Could you check a few things on this model? Use its own coordinates, in mm. A direction names the side the tool comes from. Coordinates: 2 decimals unless noted, no trailing zeros. Write each loop counter-clockwise with the first axis right and the second up, starting at its lowest first coordinate (ties: lowest second). Pieces come first, ordered by that corner, then holes. Notation, with made-up numbers: M 31,21.25 L 60,21.25 A27 ccw 60,53.25 Z; hole C 21.5,13.5 d4. An arc over 180 degrees is marked long. Answer as CSV lines item,"result". Start each with the question number.
Item 1: On a 3-axis mill with a long thin cutter (end or side, diameter ignored), from which of +Z, -Z, +X, -X, +Y, -Y can I reach the whole of each face in a straight line? I mean faces 1 (the cylindrical face through (-8.107, -8.156, 0.37)), 2 (the flat face through (8.475, 11, -4)), 3 (the cylindrical face through (6.31, 10.79, -2.46)). Say none if no direction works.
Item 2: We'd pull the mould along X, two halves only. Please class faces 4 (the flat face through (-8.475, 11, -4)), 5 (the flat face through (0, 9.45, -4)), 6 (the cylindrical face through (-8.156, 8.107, 0.37)), 7 (the cylindrical face through (-0.1, 10, 0.4)): +X half, -X half, draft (parallel to the pull), parting line (faces both ways), or undercut.
Item 3: Suppose I cut it at B-B, the plane z = -3.5. Write out the boundary of the cut face in (x, y) (3 decimals), and give its area (3 significant figures).
Item 4: I'm going to push flat-ended pins straight in: P1, Ø2, axis at x = 6.5, y = 7.5, coming from the -Z side; P2, Ø1, axis at x = 2, z = -3.5, coming from the -Y side; P3, Ø1.3, axis at y = 11, z = -3, coming from the +X side (3 decimals); P4, Ø6, axis at x = -3.5, y = -3.5, coming from the +Z side. Where does each tip first touch, or does it pass through?
Item 5: Suppose I cut it at A-A, the plane x = 0. Write out the boundary of the cut face in (y, z).
Item 6: Suppose I cut it at C-C, the plane y = 2.75. Write out the boundary of the cut face in (x, z) (3 decimals).
Item 7: If I drill on line 1 along Y through (x, z) = (0, -1); line 2 along X through (y, z) = (0, -1.2) (3 decimals); line 3 along Z through (x, y) = (6.5, 7), over which ranges is the centre line in solid material (lowest first)? Write a range as [from, to].
Item 8: Suppose I cut it at D-D, the plane z = 0.5. Write out the boundary of the cut face in (x, y) (3 decimals).
```python
from build123d import *

# Parameters (mm, degrees)
F0_W     = 20.15
F0_H     = 22.85
F1_DEPTH = 0.75
F2_W     = 20.15
F2_H     = 22.85
F2_R     = 8.5
F3_DEPTH = 2.15
F4_W     = 16.95
F4_H     = 2.65
F5_DEPTH = 3.45
F6_R     = 1.05
F7_DEPTH = 22.851


with BuildPart() as f1:
    # F0 (on Top) → F1 (new body)
    with BuildSketch(Plane.XY):
        with Locations((0, 0.675)):
            Rectangle(F0_W, F0_H)
        with BuildLine():
            ThreePointArc((8.049191, 5.933845), (9.499787, 3.123147), (10, 0))
            ThreePointArc((10, 0), (9.499787, -3.123147), (8.049191, -5.933845))
            ThreePointArc((8.049191, -5.933845), (8.43437, -6.445442), (8.571068, -7.071068))
            ThreePointArc((8.571068, -7.071068), (7.592684, -8.477452), (5.933845, -8.049191))
            ThreePointArc((5.933845, -8.049191), (0, -10), (-5.933845, -8.049191))
            ThreePointArc((-5.933845, -8.049191), (-8.131728, -8.131728), (-8.049191, -5.933845))
            ThreePointArc((-8.049191, -5.933845), (-10, 0), (-8.049191, 5.933845))
            ThreePointArc((-8.049191, 5.933845), (-8.131728, 8.131728), (-5.933845, 8.049191))
            ThreePointArc((-5.933845, 8.049191), (0, 10), (5.933845, 8.049191))
            ThreePointArc((5.933845, 8.049191), (7.592684, 8.477452), (8.571068, 7.071068))
            ThreePointArc((8.571068, 7.071068), (8.43437, 6.445442), (8.049191, 5.933845))
        make_face(mode=Mode.SUBTRACT)
    extrude(amount=F1_DEPTH)

    # F2 (on face) → F3 (join)
    with BuildSketch(Plane(origin=(0, 0, 0), x_dir=(1, 0, 0), z_dir=(0, 0, -1))):
        with Locations((0, -0.675)):
            Rectangle(F2_W, F2_H)
        Circle(F2_R, mode=Mode.SUBTRACT)
    extrude(amount=F3_DEPTH)

    # F4 (on face) → F5 (join)
    with BuildSketch(Plane(origin=(0, 0, -2.15), x_dir=(1, 0, 0), z_dir=(0, 0, -1))):
        with Locations((0, -10.775)):
            Rectangle(F4_W, F4_H)
    extrude(amount=F5_DEPTH)

    # F6 (on face) → F7 (cut, through all)
    with BuildSketch(Plane(origin=(0, 12.1, 0), x_dir=(-1, 0, 0), z_dir=(0, 1, 0))):
        with Locations((-6.175, -3.5)):
            Circle(F6_R)
        with Locations((6.175, -3.5)):
            Circle(F6_R)
    extrude(amount=-F7_DEPTH, mode=Mode.SUBTRACT)


solid = f1.part
```
Ans:
1,face 1,"+Z"
1,face 2,"-Z, +X, +Y, -Y"
1,face 3,"+Y, -Y"
2,face 4,"-X half"
2,face 5,"draft"
2,face 6,"undercut"
2,face 7,"undercut"
3,outline,"M -8.475,9.45 L -7.225,9.45 L -7.225,12.1 L -8.475,12.1 Z; M -5.125,9.45 L 5.125,9.45 L 5.125,12.1 L -5.125,12.1 Z; M 7.225,9.45 L 8.475,9.45 L 8.475,12.1 L 7.225,12.1 Z"
3,area,"33.8 mm^2"
4,P1,"stops at z = -2.15"
4,P2,"stops at y = 9.45"
4,P3,"stops at x = 8.475"
4,P4,"passes through"
5,outline,"M -10.75,-2.15 L -8.5,-2.15 L -8.5,0 L -10,0 L -10,0.75 L -10.75,0.75 Z; M 8.5,-2.15 L 9.45,-2.15 L 9.45,-5.6 L 12.1,-5.6 L 12.1,0.75 L 10,0.75 L 10,0 L 8.5,0 Z"
6,outline,"M -10.075,-2.15 L -8.043,-2.15 L -8.043,0 L -9.614,0 L -9.614,0.75 L -10.075,0.75 Z; M 8.043,-2.15 L 10.075,-2.15 L 10.075,0.75 L 9.614,0.75 L 9.614,0 L 8.043,0 Z"
7,line 1,"y = [-10.75, -8.5], [8.5, 12.1]"
7,line 2,"x = [-10.075, -8.5], [8.5, 10.075]"
7,line 3,"z = [-2.15, 0]"
8,outline,"M -10.075,-10.75 L 10.075,-10.75 L 10.075,12.1 L -10.075,12.1 Z; hole M -8.049,-5.934 A1.5 ccw long -5.934,-8.049 A10 ccw 5.934,-8.049 A1.5 ccw long 8.049,-5.934 A10 ccw 10,0 A10 ccw 8.049,5.934 A1.5 ccw long 5.934,8.049 A10 ccw -5.934,8.049 A1.5 ccw long -8.049,5.934 A10 ccw Z"
